Could you check a few things on this model? Use its own coordinates, in mm. A direction names the side the tool comes from. Give positions to 0.01 mm unless a question says otherwise; leave off trailing zeros. Write each loop counter-clockwise with the first axis right and the second up, starting at its lowest first coordinate (ties: lowest second). Pieces come first, ordered by that corner, then holes. Notation, with made-up numbers: (-34, -6.75) - (-27, -6.75) arc R26 cw to (-27, 30.25) - close; hole circle Ø5 at (-2.5, 86). An arc over 180 degrees is marked (long way). Use one line per item in the form item = value.
Autodesk Inventor part; units mm, degrees
ref_plane "YZ Plane" through (0, 0, 0) normal (1, 0, 0) x (0, 1, 0)
ref_plane "XZ Plane" through (0, 0, 0) normal (0, 1, 0) x (-1, 0, 0)
ref_plane "XY Plane" through (0, 0, 0) normal (0, 0, 1) x (1, 0, 0)
sketch "Sketch1" plane through (0, 0, 0) normal (0, 1, 0) x (-1, 0, 0)
  line L0 (0, 0) -> (9, 0)
  line L1 (9, 0) -> (9, -12.5)
  line L2 (9, -12.5) -> (2.5, -12.5)
  circle A0 centre (2.5, -15) radius 2.5
  circle A1 centre (2.5, -15) radius 1
  line L3 (2.5, -15) -> (17.5, -15) construction
  circle A2 centre (6, -25.188) radius 3
  circle A3 centre (6, -25.188) radius 1
  line L4 (0, -15.4175) -> (3.0968, -24.4319)
  line L5 (9, 0) -> (17.3, 0)
  line L6 (17.3, 0) -> (17.3, -8)
  line L7 (17.3, -8) -> (27.3459, -13.8)
  line L8 (27.3459, -13.8) -> (27.3459, 0)
  line L9 (30.3459, 0) -> (30.3459, -15.6149)
  line L10 (30.3459, -15.6149) -> (37.3459, -39.6149)
  line L11 (37.3459, -39.6149) -> (37.3459, -49.6149)
  line L12 (29.6459, -39.6149) -> (29.6459, -49.6149)
  line L13 (37.3459, -49.6149) -> (29.6459, -49.6149)
  line L14 (29.6459, -39.6149) -> (80.5305, -39.6149) construction
  arc A4 (14.4139, -18.9731) -> (9, -20.7544) centre (12, -20.7544) ccw
  line L15 (29.6459, -39.6149) -> (19, -25.188)
  line L16 (19, -25.188) -> (16.5834, -21.9131)
  line L17 (16.5834, -21.9131) -> (14.4139, -18.9731)
  line L18 (9, -20.7544) -> (9, -25.188)
  circle A5 centre (12, -7) radius 1
  circle A6 centre (34.3459, -39.6149) radius 3
  circle A7 centre (34.3459, -39.6149) radius 1
  line L19 (30.3459, 0) -> (0, 0)
  line L20 (9, 0) -> (9, 12.5)
  line L21 (9, 12.5) -> (2.5, 12.5)
  circle A8 centre (2.5, 15) radius 2.5
  circle A9 centre (2.5, 15) radius 1
  line L22 (2.5, 15) -> (17.5, 15) construction
  circle A10 centre (6, 25.188) radius 3
  circle A11 centre (6, 25.188) radius 1
  line L23 (0, 15.4175) -> (3.0968, 24.4319)
  line L24 (17.3, 0) -> (17.3, 8)
  line L25 (17.3, 8) -> (27.3459, 13.8)
  line L26 (27.3459, 13.8) -> (27.3459, 0)
  line L27 (30.3459, 0) -> (30.3459, 15.6149)
  line L28 (30.3459, 15.6149) -> (37.3459, 39.6149)
  line L29 (37.3459, 39.6149) -> (37.3459, 49.6149)
  line L30 (29.6459, 39.6149) -> (29.6459, 49.6149)
  line L31 (37.3459, 49.6149) -> (29.6459, 49.6149)
  line L32 (29.6459, 39.6149) -> (80.5305, 39.6149) construction
  arc A12 (9, 20.7544) -> (14.4139, 18.9731) centre (12, 20.7544) ccw
  line L33 (29.6459, 39.6149) -> (19, 25.188)
  line L34 (19, 25.188) -> (16.5834, 21.9131)
  line L35 (16.5834, 21.9131) -> (14.4139, 18.9731)
  line L36 (9, 20.7544) -> (9, 25.188)
  circle A13 centre (12, 7) radius 1
  circle A14 centre (34.3459, 39.6149) radius 3
  circle A15 centre (34.3459, 39.6149) radius 1
  arc A16 (12, -9) -> (12, -5) centre (12, -7) ccw
  arc A17 (12, 5) -> (12, 9) centre (12, 7) ccw
  line L37 (12, 5) -> (9, 5)
  line L38 (12, 9) -> (9, 9)
  line L39 (12, -5) -> (9, -5)
  line L40 (12, -9) -> (9, -9)
  point P0 (0.1356, 15.8123)
  point P1 (0.1356, -15.8123)
  point P2 (36.8755, -38.0021)
  dimension "d3" = 5
  dimension "d0" = 9
  dimension "d1" = 12.5
  dimension "d4" = 2
  dimension "d7" = 6
  dimension "d9" = 2
  dimension "d13" = 8.3
  dimension "d14" = 8
  dimension "d15" = 11.6
  dimension "d16" = 120
  dimension "d17" = 3
  dimension "d20" = 7.7
  dimension "d21" = 10
  dimension "d23" = 6
  dimension "d24" = 10
  dimension "d27" = 2
  dimension "d28" = 7
  dimension "d29" = 6
  dimension "d30" = 2
  dimension "d31" = 4
  dimension "d32" = 4
extrude "Extrusion1" add sketch "Sketch1" along normal blind 5 contours L5 L6 L7 L8 L19 L9 L10 A6 L11 L13 L12 L15 L16 L17 A4 L18 A2 L4 A0 L2 L1 L40 A16 L39 | L20 L37 A17 L38 L21 A8 L23 A10 L36 A12 L35 L34 L33 L30 L31 L29 A14 L28 L27 L19 L26 L25 L24 L5 | L39 A16 L40 L1 | L20 L38 A17 L37 | A0 | A8 | L10 A6 | A14 L28 | A2 | A10 picked at (36.5127, -38.9975) picked at (36.5127, 38.9975)
extrude "Extrusion2" cut sketch "Sketch1" along normal blind 2 contours L39 A16 L40 L1 | L20 L38 A17 L37 | A0 | A8
extrude "Extrusion3" add sketch "Sketch1" against normal blind 2 contours A2 | A10
sketch "Sketch2" plane through (0, 5, 0) normal (0, 1, 0) x (1, 0, 0)
  circle A0 centre (-34.3459, 39.6149) radius 1
  line L0 (-37.3459, 49.6149) -> (-37.3459, 39.6149)
  circle A1 centre (-34.3459, 39.6149) radius 3
  circle A2 centre (-34.3459, -39.6149) radius 1
  circle A3 centre (-34.3459, -39.6149) radius 3
  line L1 (-37.3459, -39.6149) -> (-37.3459, -49.6149)
  line L2 (-37.3459, -39.6149) -> (-37.3459, -49.6149)
  line L3 (-37.3459, -49.6149) -> (-29.6459, -49.6149)
  line L4 (-37.3459, -49.6149) -> (-29.6459, -49.6149)
  line L5 (-29.6459, -49.6149) -> (-29.6459, -39.6149)
  line L6 (-29.6459, -49.6149) -> (-29.6459, -39.6149)
  line L7 (-29.6459, -39.6149) -> (-31.3459, -39.6149)
  line L8 (-37.3459, 39.6149) -> (-37.3459, 49.6149)
  line L9 (-37.3459, 49.6149) -> (-29.6459, 49.6149)
  line L10 (-29.6459, 49.6149) -> (-29.6459, 39.6149)
  line L11 (-29.6459, 39.6149) -> (-31.3459, 39.6149)
  point P0 (0, 0)
extrude "Extrusion5" add sketch "Sketch2" along normal blind 10 contours A1 | A3
extrude "Extrusion6" add sketch "Sketch2" along normal blind 3 contours L9 L10 L11 A1 L0 | L7 L5 L3 L1 A3
sketch "Sketch3" plane through (-37.3459, 0, 39.6149) normal (-1, 0, 0) x (0, 0, 1)
  circle A0 centre (5, 4) radius 2
  line L0 (10, 0) -> (10, 8)
  arc A1 (2, 0) -> (2, 8) centre (5, 4) ccw
  circle A2 centre (-84.2298, 4) radius 2
  line L1 (-89.2298, 0) -> (-89.2298, 8)
  arc A3 (-81.2298, 8) -> (-81.2298, 0) centre (-84.2298, 4) ccw
  line L2 (-89.2298, 0) -> (-79.2298, 0)
  line L3 (-87.2298, 0) -> (-89.2298, 0)
  line L4 (-89.2298, 0) -> (-89.2298, 8)
  line L5 (-89.2298, 0) -> (-89.2298, 8)
  line L6 (-89.2298, 8) -> (-87.2298, 8)
  line L7 (-79.2298, 8) -> (-89.2298, 8)
  arc A4 (-87.2298, 8) -> (-87.2298, 0) centre (-84.2298, 4) ccw
  line L8 (0, 0) -> (10, 0)
  line L9 (10, 8) -> (0, 8)
  arc A5 (8, 0) -> (8, 8) centre (5, 4) ccw
  line L10 (8, 0) -> (10, 0)
  line L11 (10, 8) -> (8, 8)
  point P0 (-39.6149, 0)
  point P1 (10, 4)
  point P2 (-89.2298, 4)
  dimension "d45" = 4
  dimension "d46" = 5
  dimension "d47" = 4
  dimension "d48" = 5
extrude "Extrusion7" add sketch "Sketch3" against normal blind 7.7 contours A1 L8 | L9 A1 | A3 L7 | L2 A3
extrude "Extrusion8" cut sketch "Sketch3" against normal blind 10 contours A0 | L8 A1 L0 | A1 L9 L0 | A2 | L1 L6 A3 | L1 A3 L2
properties part number "PX9200-11"
1. Imagine slicing it at A-A, the plane z = 7. List the corners of the cut face in (x, y) for me, and give its area (3 significant figures).
Response values:
outline = (-30.35, 0) - (-27.35, 0) - (-27.35, 5) - (-30.35, 5) - close; (-17.3, 0) - (-14, 0) - (-14, 2) - (-13, 2) - (-13, 5) - (-17.3, 5) - close; (-11, 2) - (-9, 2) - (-9, 5) - (-11, 5) - close
area = 40.5 mm²
2. Imagine slicing it at C-C, the plane x = -21.5. List the corners of the cut face in (y, z) for me, and give its area (3 significant figures).
Response values:
outline = (0, -28.58) - (5, -28.58) - (5, -10.42) - (0, -10.42) - close; (0, 10.42) - (5, 10.42) - (5, 28.58) - (0, 28.58) - close
area = 182 mm²
3. Imagine slicing it at B-B, the plane x = -6. List the corners of the cut face in (y, z) for me, and give its area (3 significant figures).
Response values:
outline = (-2, -28.19) - (5, -28.19) - (5, -26.19) - (-2, -26.19) - close; (-2, -24.19) - (5, -24.19) - (5, -12.5) - (0, -12.5) - (0, -22.19) - (-2, -22.19) - close; (-2, 22.19) - (0, 22.19) - (0, 12.5) - (5, 12.5) - (5, 24.19) - (-2, 24.19) - close; (-2, 26.19) - (5, 26.19) - (5, 28.19) - (-2, 28.19) - close
area = 153 mm²
4. Imagine slicing it at D-D, the plane x = -28.5. List the corners of the cut face in (y, z) for me, and give its area (3 significant figures).
Response values:
outline = (0, -38.06) - (5, -38.06) - (5, 38.06) - (0, 38.06) - close
area = 381 mm²
5. If we mould it in two halves opening along Z, with no side actions, what happens to faces 6 (the face through (-11.11, 2.46, 17.89)), 7 (the face through (-29.646, 6.2, -44.5)), 8 (the face through (-11.263, 3.479, -7.676))? For each: pulls with the +Z half, pulls with the -Z half, needs draft (parallel to the pull), parting line crosses it, or undercut.
Response values:
face_6 = pulls with the +Z half
face_7 = needs draft
face_8 = undercut
6. For pin 1 (2 mm diameter, centred on y = 2, z = -31.5, fed in from +X); pin 2 (6 mm diameter, centred on x = -31, y = 3, fed in from -Z); pin 3 (5 mm diameter, centred on x = -11.5, z = 18, fed in from -Y); pin 4 (1.6 mm diameter, centred on x = -10.5, y = 1, fed in from +Z), each with a flat end and sliding along its axis, tell me the tip position at first contact or that it passes through.
Response values:
pin_1 = -22.92
pin_2 = -49.61
pin_3 = 0
pin_4 = 18.83
7. If I drill on line 1 (X direction, y = 2.25, z = 3); line 2 (Z direction, x = -6, y = 2.5); line 3 (Z direction, x = -12, y = 3.4), over which ranges is the centre line in solid material (lowest first)? Write a range as from..to.
Response values:
line_1 = -30.35..-27.35, -17.3..-9
line_2 = -28.19..-26.19, -24.19..-12.5, 12.5..24.19, 26.19..28.19
line_3 = -17.75..-8, -6..6, 8..17.75
8. Which directions (+Z, -Z, +X, -X, +Y, -Y) give clear straight access to the entire face, cutting with the end or side of a thin tool? Please do faces 1 (the face through (-29.646, 6.2, 44.5)), 2 (the face through (-6, 2, -12.5)), 3 (the face through (-10.9, 2, 7.5)), 4 (the face through (-9, 2, 23)), 5 (the face through (-5.609, 0.771, 28.162)).
Response values:
face_1 = +Z, +X, +Y, -Y
face_2 = +X, +Y, -Y
face_3 = +X, -Y
face_4 = +Z, +Y, -Y
face_5 = -Y
